```python
from build123d import *

# Parameters (mm, degrees)
SKETCH_1_R       = 5
EXTRUDE_1_DEPTH  = 52
SKETCH_2_R       = 3.5
EXTRUDE_2_DEPTH  = 2
SKETCH_3_R       = 5
EXTRUDE_3_DEPTH  = 14
SKETCH_4_R       = 3.5
EXTRUDE_4_DEPTH  = 2
SKETCH_5_R       = 5
EXTRUDE_5_DEPTH  = 4
SKETCH_6_R       = 3.5
EXTRUDE_6_DEPTH  = 2
SKETCH_7_R       = 5
EXTRUDE_7_DEPTH  = 10
EXTRUDE_START    = 2
SKETCH_8_R       = 3.5
EXTRUDE_8_DEPTH  = 2
EXTRUDE_START_2  = 14
SKETCH_9_R       = 5
EXTRUDE_9_DEPTH  = 14
SKETCH_10_R      = 3.5
EXTRUDE_10_DEPTH = 2
EXTRUDE_START_3  = 4
SKETCH_11_R      = 5
EXTRUDE_11_DEPTH = 4
SKETCH_12_R      = 3.5
EXTRUDE_12_DEPTH = 2
EXTRUDE_START_4  = 10
SKETCH_13_R      = 5
EXTRUDE_13_DEPTH = 10
CHAMFER_1_SIZE   = 0.5


with BuildPart() as part:
    # 草图1 → 凸台-拉伸1 (new body)
    with BuildSketch(Plane(origin=(0, 0, 0), x_dir=(0, 0, -1), z_dir=(1, 0, 0))):
        with Locations(Location((0, 0, 0), (0, 0, 180))):
            Circle(SKETCH_1_R)
    extrude(amount=EXTRUDE_1_DEPTH)

    # 草图2 → 凸台-拉伸2 (add)
    with BuildSketch(Plane(origin=(52, 0, 0), x_dir=(0, 0, -1), z_dir=(1, 0, 0))):
        Circle(SKETCH_2_R)
    extrude(amount=EXTRUDE_2_DEPTH)

    # 草图3 → 凸台-拉伸3 (add)
    with BuildSketch(Plane(origin=(54, 0, 0), x_dir=(0, 0, -1), z_dir=(1, 0, 0))):
        with Locations(Location((0, 0, 0), (0, 0, 180))):
            Circle(SKETCH_3_R)
    extrude(amount=EXTRUDE_3_DEPTH)

    # 草图4 → 凸台-拉伸4 (add)
    with BuildSketch(Plane(origin=(68, 0, 0), x_dir=(0, 0, -1), z_dir=(1, 0, 0))):
        Circle(SKETCH_4_R)
    extrude(amount=EXTRUDE_4_DEPTH)

    # 草图5 → 凸台-拉伸5 (add)
    with BuildSketch(Plane(origin=(70, 0, 0), x_dir=(0, 0, -1), z_dir=(1, 0, 0))):
        with Locations(Location((0, 0, 0), (0, 0, 180))):
            Circle(SKETCH_5_R)
    extrude(amount=EXTRUDE_5_DEPTH)

    # 草图6 → 凸台-拉伸6 (add)
    with BuildSketch(Plane(origin=(74, 0, 0), x_dir=(0, 0, -1), z_dir=(1, 0, 0))):
        Circle(SKETCH_6_R)
    extrude(amount=EXTRUDE_6_DEPTH)

    # 草图7 → 凸台-拉伸7 (add)
    with BuildSketch(Plane(origin=(76, 0, 0), x_dir=(0, 0, -1), z_dir=(1, 0, 0))):
        with Locations(Location((0, 0, 0), (0, 0, 180))):
            Circle(SKETCH_7_R)
    extrude(amount=EXTRUDE_7_DEPTH)

    # 草图8 → 凸台-拉伸8 (add)
    with BuildSketch(Plane.ZY.offset(EXTRUDE_START)):
        with Locations(Location((0, 0, 0), (0, 0, 180))):
            Circle(SKETCH_8_R)
    extrude(amount=-EXTRUDE_8_DEPTH)

    # 草图9 → 凸台-拉伸9 (add)
    with BuildSketch(Plane.ZY.offset(2).offset(EXTRUDE_START_2)):
        Circle(SKETCH_9_R)
    extrude(amount=-EXTRUDE_9_DEPTH)

    # 草图10 → 凸台-拉伸10 (add)
    with BuildSketch(Plane.ZY.offset(16).offset(EXTRUDE_START)):
        with Locations(Location((0, 0, 0), (0, 0, 180))):
            Circle(SKETCH_10_R)
    extrude(amount=-EXTRUDE_10_DEPTH)

    # 草图11 → 凸台-拉伸11 (add)
    with BuildSketch(Plane.ZY.offset(18).offset(EXTRUDE_START_3)):
        Circle(SKETCH_11_R)
    extrude(amount=-EXTRUDE_11_DEPTH)

    # 草图12 → 凸台-拉伸12 (add)
    with BuildSketch(Plane.ZY.offset(22).offset(EXTRUDE_START)):
        with Locations(Location((0, 0, 0), (0, 0, 180))):
            Circle(SKETCH_12_R)
    extrude(amount=-EXTRUDE_12_DEPTH)

    # 草图13 → 凸台-拉伸13 (add)
    with BuildSketch(Plane.ZY.offset(24).offset(EXTRUDE_START_4)):
        Circle(SKETCH_13_R)
    extrude(amount=-EXTRUDE_13_DEPTH)

    # 倒角1
    chamfer_1_edges = [part.edges().sort_by_distance(p)[0] for p in [
        (86, 0, -5),
        (-34, 0, -5),
    ]]
    chamfer(chamfer_1_edges, length=CHAMFER_1_SIZE)


solid = part.part
```
Read the model definition and answer for the solid it produces. Units are mm, in the model's axes. A direction names the side the tool comes from. Coordinates: 2 decimals unless noted, no trailing zeros. Write each loop counter-clockwise with the first axis right and the second up, starting at its lowest first coordinate (ties: lowest second). Pieces come first, ordered by that corner, then holes. Notation, with made-up numbers: (59.25, 64.25) -> (114.25, 64.25) arc R19 cw to (114.25, 101.25) -> close; hole circle Ø7 at (17, -2.75). An arc over 180 degrees is marked (long way). Answer as a JSON object with one key per item and string values.
Q1. The part is cut by section A-A on x = -20. Give the vertices of the cut face in (y, z).
The answers:
{"outline": "circle Ø10 at (0, 0)"}
Q2. Consider line 1 (Z direction, x = 11.5, y = 0.25); line 2 (Y direction, x = 47.5, z = -3.5). Determine where each line is inside the solid, lowest interval first. Write a range as [from, to].
The answers:
{"line 1": "z = [-4.99, 4.99]", "line 2": "y = [-3.57, 3.57]"}
Q3. A tool of negligible diameter and unlimited length cuts with its end or side. For faces 1 (the flat face through (74, 2.2, 3.3)), 2 (the cylindrical face through (-28.82, -4.88, -1.08)), from which of +Z, -Z, +X, -X, +Y, -Y can it reach the whole face along a straight path? Write none if from no direction.
The answers:
{"face 1": "none", "face 2": "+X, -X"}
Q4. Determine the mould class of faces 3 (the flat face through (86, 0, 0)), 4 (the cylindrical face through (-17.014, 1.341, -3.233)), 5 (the flat face through (-34, 0, 0)) for opening direction X: pulls with the +X half, pulls with the -X half, needs draft (parallel to the pull), parting line crosses it, or undercut.
The answers:
{"face 3": "pulls with the +X half", "face 4": "undercut", "face 5": "pulls with the -X half"}
Q5. Flat-ended cylindrical pins translate along their axes: pin 1 Ø1.5 at (x, z) = (17.5, 1.5) entering from -Y; pin 2 Ø1 at (x, y) = (44, 2) entering from +Z; pin 3 Ø5 at (x, y) = (30, -2.5) entering from +Z; pin 4 Ø5 at (x, z) = (59.5, -3) entering from +Y. Find the tip coordinate at first contact, or state that the pin passes through.
The answers:
{"pin 1": "stops at y = -4.94", "pin 2": "stops at z = 4.77", "pin 3": "stops at z = 5", "pin 4": "stops at y = 4.97"}
